Geometry check sheet. Reference: the model listing, model coordinates, mm. Face numbers are marked on the shaded views. A direction names the side the tool comes from. Coordinates: 2 decimals unless noted, no trailing zeros. Order: outer loops, then holes, each group sorted by start corner. A loop starts at its lowest first (then second) coordinate and runs counter-clockwise, first axis right, second up. Notation, with made-up numbers: M -2.5,-23.75 L 26.5,-23.75 A24 cw 26.5,-1.75 Z; hole C -28,-9.75 d8. An arc over 180 degrees is marked long. One line per item, written item: value. Start each with the question number.
1) Access from +Z, -Z, +X, -X, +Y, -Y to the whole of each face (thin tool, end or side, straight path). Record for the marked faces 1, 2 and 3.
2) Thickness scan on L1, parallel to Y at x = 21, z = 23; L2, parallel to X at y = 23.5, z = 14; L3, parallel to Y at x = 57, z = 28. Record the ranges inside material, lowest first. Write a range as from..to.
3) Sectioned sample at B-B, the plane y = 13.5. Enter the section's corners in (x, z), then the cut area to 3 significant figures.
4) Go/stop test with flat-tipped pins: P1, Ø1.5, axis at y = -4, z = 31, coming from the -X side; P2, Ø5, axis at x = 71.5, y = -8.5, coming from the +Z side; P3, Ø8, axis at x = 39, z = 19.5, coming from the -Y side. Record where each tip stops, or that it passes through.
5) Sectioned sample at A-A, the plane x = 39. Enter the section's corners in (y, z), then the cut area to 3 significant figures.
6) Sectioned sample at C-C, the plane x = 87. Enter the section's corners in (y, z).
7) Sectioned sample at D-D, the plane x = 16.5. Enter the section's corners in (y, z), then the cut area to 3 significant figures.
8) Draft check along Y on the marked faces 4, 5, 6 and 7. Enter one of: pulls with the +Y half, pulls with the -Y half, needs draft (parallel to the pull), parting line crosses it, or undercut.
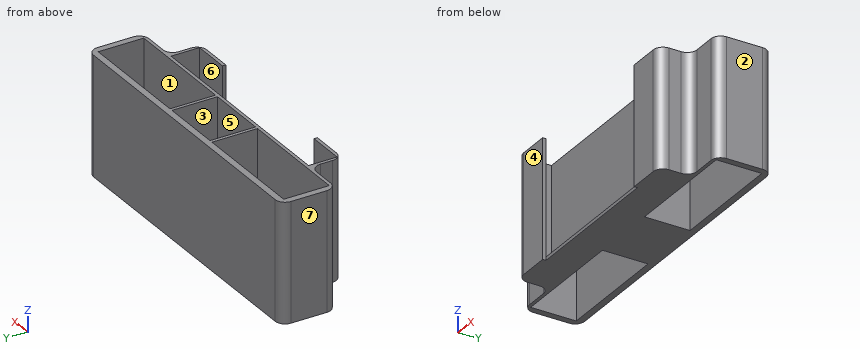
```python
from build123d import *

# Parameters (mm, degrees)
SKETCH2_W            = 141.5
SKETCH2_H            = 21.5
BOSS_EXTRUDE1_DEPTH  = 73
SHELL1_T             = -2
CUT_EXTRUDE1_REACH   = 162.666
SKETCH3_W            = 91.5
SKETCH3_H            = 2
SKETCH7_W            = 73
SKETCH7_H            = 2
BOSS_EXTRUDE5_DEPTH  = 26
SKETCH8_W            = 73
SKETCH8_H            = 2
BOSS_EXTRUDE6_DEPTH  = 26
SKETCH9_W            = 4
SKETCH9_H            = 73
BOSS_EXTRUDE7_DEPTH  = 28
SKETCH10_W           = 193.5
SKETCH10_H           = 73
BOSS_EXTRUDE8_DEPTH  = 4
SKETCH11_W           = 2
SKETCH11_H           = 73
BOSS_EXTRUDE9_DEPTH  = 28
SKETCH13_W           = 38
SKETCH13_H           = 2
BOSS_EXTRUDE10_DEPTH = 28
FILLET1_R            = 6


with BuildPart() as part:
    # Sketch2 → Boss-Extrude1 (new body)
    with BuildSketch(Plane.XY):
        with Locations((70.75, -10.75)):
            Rectangle(SKETCH2_W, SKETCH2_H)
    extrude(amount=BOSS_EXTRUDE1_DEPTH)

    # Shell1
    shell1_openings = [part.faces().sort_by_distance(p)[0] for p in [
        (70.75, -10.75, 73),
    ]]
    offset(amount=SHELL1_T, openings=shell1_openings, kind=Kind.INTERSECTION)

    # Cut-Extrude1: up to this face of the body (flat: up to its plane)
    cut_extrude1_end = Plane(part.part.faces().sort_by_distance((70.75, -10.75, 0))[0])
    # Sketch3 → Cut-Extrude1 (cut, up to the picked face)
    with BuildSketch(Plane.XY.offset(73), mode=Mode.PRIVATE) as cut_extrude1_sk1:
        with Locations((70.75, -20.5)):
            Rectangle(SKETCH3_W, SKETCH3_H)
    cut_extrude1_tool1 = split(extrude(cut_extrude1_sk1.sketch, amount=-CUT_EXTRUDE1_REACH, mode=Mode.PRIVATE), bisect_by=cut_extrude1_end, keep=Keep.BOTH, mode=Mode.PRIVATE)
    add(cut_extrude1_tool1.solids().sort_by(Axis((70.75, -20.5, 73), (0, 0, -1)))[0], mode=Mode.SUBTRACT)

    # Sketch7 → Boss-Extrude5 (add)
    with BuildSketch(Plane.ZY):
        with Locations((36.5, -1)):
            Rectangle(SKETCH7_W, SKETCH7_H)
    extrude(amount=BOSS_EXTRUDE5_DEPTH)

    # Sketch8 → Boss-Extrude6 (add)
    with BuildSketch(Plane(origin=(141.5, 0, 0), x_dir=(0, 0, -1), z_dir=(1, 0, 0))):
        with Locations((-36.5, -1)):
            Rectangle(SKETCH8_W, SKETCH8_H)
    extrude(amount=BOSS_EXTRUDE6_DEPTH)

    # Sketch9 → Boss-Extrude7 (add)
    with BuildSketch(Plane(origin=(0, 0, 0), x_dir=(1, 0, 0), z_dir=(0, 1, 0))):
        with Locations((165.5, -36.5)):
            Rectangle(SKETCH9_W, SKETCH9_H)
        with Locations((-24, -36.5)):
            Rectangle(SKETCH9_W, SKETCH9_H)
    extrude(amount=BOSS_EXTRUDE7_DEPTH)

    # Sketch10 → Boss-Extrude8 (add)
    with BuildSketch(Plane(origin=(0, 28, 0), x_dir=(1, 0, 0), z_dir=(0, 1, 0))):
        with Locations((70.75, -36.5)):
            Rectangle(SKETCH10_W, SKETCH10_H)
    extrude(amount=BOSS_EXTRUDE8_DEPTH)

    # Sketch11 → Boss-Extrude9 (add)
    with BuildSketch(Plane(origin=(0, 0, 0), x_dir=(1, 0, 0), z_dir=(0, 1, 0))):
        with Locations((50.75, -36.5)):
            Rectangle(SKETCH11_W, SKETCH11_H)
        with Locations((90.75, -36.5)):
            Rectangle(SKETCH11_W, SKETCH11_H)
    extrude(amount=BOSS_EXTRUDE9_DEPTH)

    # Sketch13 → Boss-Extrude10 (add)
    with BuildSketch(Plane(origin=(0, 0, 0), x_dir=(1, 0, 0), z_dir=(0, 1, 0))):
        with Locations((70.75, -1)):
            Rectangle(SKETCH13_W, SKETCH13_H)
    extrude(amount=BOSS_EXTRUDE10_DEPTH)

    # Fillet1
    fillet1_edges = [part.edges().sort_by_distance(p)[0] for p in [
        (167.5, 32, 36.5),
        (0, -2, 36.5),
        (-26, -2, 36.5),
        (141.5, -2, 36.5),
        (167.5, -2, 36.5),
        (141.5, -21.5, 36.5),
        (0, -21.5, 36.5),
        (-26, 32, 36.5),
    ]]
    fillet(fillet1_edges, radius=FILLET1_R)


solid = part.part
```
Final values:
1. face 1: +Z, -Z
1. face 2: +Z, -Z, +X, +Y, -Y
1. face 3: +Z
2. L1: y = -21.5..-19.5, -2..0, 28..32
2. L2: x = -26..-22, 49.75..51.75, 89.75..91.75, 163.5..167.5
2. L3: y = -2..0, 28..32
3. outline: M -26,0 L -22,0 L -22,73 L -26,73 Z; M 49.75,0 L 91.75,0 L 91.75,73 L 89.75,73 L 89.75,2 L 51.75,2 L 51.75,73 L 49.75,73 Z; M 163.5,0 L 167.5,0 L 167.5,73 L 163.5,73 Z
3. area: 952 mm^2
4. P1: stops at x = -2.33
4. P2: stops at z = 2
4. P3: stops at y = -2
5. outline: M -19.5,0 L 0,0 L 0,73 L -2,73 L -2,2 L -19.5,2 Z; M 28,0 L 32,0 L 32,73 L 28,73 Z
5. area: 473 mm^2
6. outline: M -19.5,0 L 32,0 L 32,73 L 28,73 L 28,2 L 0,2 L 0,73 L -2,73 L -2,2 L -19.5,2 Z
7. outline: M -21.5,0 L 0,0 L 0,73 L -2,73 L -2,2 L -19.5,2 L -19.5,73 L -21.5,73 Z; M 28,0 L 32,0 L 32,73 L 28,73 Z
7. area: 619 mm^2
8. face 4: pulls with the -Y half
8. face 5: undercut
8. face 6: undercut
8. face 7: needs draft
